from build123d import *

# Parameters (mm, degrees)
BOSS_EXTRUDE1_DEPTH = 5
SKETCH2_W           = 24.8
SKETCH2_H           = 23.2
CUT_EXTRUDE1_DEPTH  = 5
BOSS_EXTRUDE2_START = 5
BOSS_EXTRUDE2_DEPTH = 5
SKETCH4_R           = 1.95
CUT_EXTRUDE2_DEPTH  = 10
CUT_EXTRUDE3_DEPTH  = 5
CUT_EXTRUDE4_DEPTH  = 29.2


with BuildPart() as part:
    # Sketch1 → Boss-Extrude1 (new body)
    with BuildSketch(Plane.XY):
        with BuildLine():
            Line((14.2, 0), (14.2, 5))
            Line((14.2, 5), (50, 5))
            Line((50, 5), (50, -24.2))
            Line((50, -24.2), (-50, -24.2))
            Line((-50, -24.2), (-50, 5))
            Line((-50, 5), (-14.2, 5))
            Line((-14.2, 5), (-14.2, 0))
            ThreePointArc((-14.2, 0), (0, -14.2), (14.2, 0))
        make_face()
        with BuildLine():
            Line((-5, -18.431553888), (5, -18.431553888))
            ThreePointArc((5, -18.431553888), (7, -20.431553888), (5, -22.431553888))
            Line((5, -22.431553888), (-5, -22.431553888))
            ThreePointArc((-5, -22.431553888), (-7, -20.431553888), (-5, -18.431553888))
        make_face(mode=Mode.SUBTRACT)
    extrude(amount=BOSS_EXTRUDE1_DEPTH)

    # Sketch2 → Cut-Extrude1 (cut)
    with BuildSketch(Plane.XY.offset(5)):
        with Locations((-33.6, -9.6)):
            Rectangle(SKETCH2_W, SKETCH2_H)
        with Locations((33.6, -9.6)):
            Rectangle(SKETCH2_W, SKETCH2_H)
    extrude(amount=-CUT_EXTRUDE1_DEPTH, mode=Mode.SUBTRACT)

    # Sketch3 → Boss-Extrude2 (add)
    with BuildSketch(Plane(origin=(0, 0, 0), x_dir=(-1, 0, 0), z_dir=(0, 0, -1)).offset(BOSS_EXTRUDE2_START)):
        with BuildLine():
            Line((-20, 5), (-20, 0))
            ThreePointArc((-20, 0), (-19.267766953, -1.767766953), (-17.5, -2.5))
            Line((-17.5, -2.5), (-13.978197309, -2.5))
            ThreePointArc((-13.978197309, -2.5), (-14.144440636, -1.25491), (-14.2, 0))
            Line((-14.2, 0), (-14.2, 5))
            Line((-14.2, 5), (-20, 5))
        make_face()
        with BuildLine():
            ThreePointArc((14.2, 0), (14.144440636, -1.25491), (13.978197309, -2.5))
            Line((13.978197309, -2.5), (17.5, -2.5))
            ThreePointArc((17.5, -2.5), (19.267766953, -1.767766953), (20, 0))
            Line((20, 0), (20, 5))
            Line((20, 5), (14.2, 5))
            Line((14.2, 5), (14.2, 0))
        make_face()
    extrude(amount=-BOSS_EXTRUDE2_DEPTH)

    # Sketch4 → Cut-Extrude2 (cut)
    with BuildSketch(Plane(origin=(0, 0, -5), x_dir=(-1, 0, 0), z_dir=(0, 0, -1))):
        with Locations((-17.5, 0)):
            Circle(SKETCH4_R)
        with Locations((17.5, 0)):
            Circle(SKETCH4_R)
    extrude(amount=-CUT_EXTRUDE2_DEPTH, mode=Mode.SUBTRACT)

    # Sketch5 → Cut-Extrude3 (cut)
    with BuildSketch(Plane.XY.offset(5)):
        with BuildLine():
            Line((-7.5, -15.547171584), (-7.5, -13.852075657))
            ThreePointArc((-7.5, -13.852075657), (-7.513947323, -13.801135135), (-7.551898734, -13.764404292))
            ThreePointArc((-7.551898734, -13.764404292), (-8.068261954, -13.46822739), (-8.573026316, -13.15268869))
            ThreePointArc((-8.573026316, -13.15268869), (-8.739609576, -12.972022031), (-8.8, -12.733813254))
            Line((-8.8, -12.733813254), (-8.8, -11.099557513))
            Line((-8.8, -11.099557513), (8.8, -11.099557513))
            Line((8.8, -11.099557513), (8.8, -12.733813254))
            ThreePointArc((8.8, -12.733813254), (8.739609576, -12.972022031), (8.573026316, -13.15268869))
            ThreePointArc((8.573026316, -13.15268869), (8.068261954, -13.46822739), (7.551898734, -13.764404292))
            ThreePointArc((7.551898734, -13.764404292), (7.513947323, -13.801135135), (7.5, -13.852075657))
            Line((7.5, -13.852075657), (7.5, -15.547171584))
            ThreePointArc((7.5, -15.547171584), (7.148528137, -16.395699721), (6.3, -16.747171584))
            Line((6.3, -16.747171584), (-6.3, -16.747171584))
            ThreePointArc((-6.3, -16.747171584), (-7.148528137, -16.395699721), (-7.5, -15.547171584))
        make_face()
    extrude(amount=-CUT_EXTRUDE3_DEPTH, mode=Mode.SUBTRACT)

    # Sketch7 → Cut-Extrude4 (cut)
    with BuildSketch(Plane(origin=(0, 5, 0), x_dir=(1, 0, 0), z_dir=(0, 1, 0))):
        with BuildLine():
            Line((49.696579359, 0), (50, 0))
            Line((50, 0), (50, -5))
            Line((50, -5), (49.997973832, -5.049874854))
            ThreePointArc((49.997973832, -5.049874854), (49.911184048, -2.521123203), (49.696579359, 0))
        make_face()
        with BuildLine():
            Line((-50, -5), (-49.997973832, -5.049874854))
            ThreePointArc((-49.997973832, -5.049874854), (-49.911184048, -2.521123203), (-49.696579359, 0))
            Line((-49.696579359, 0), (-50, 0))
            Line((-50, 0), (-50, -5))
        make_face()
    extrude(amount=-CUT_EXTRUDE4_DEPTH, mode=Mode.SUBTRACT)


solid = part.part
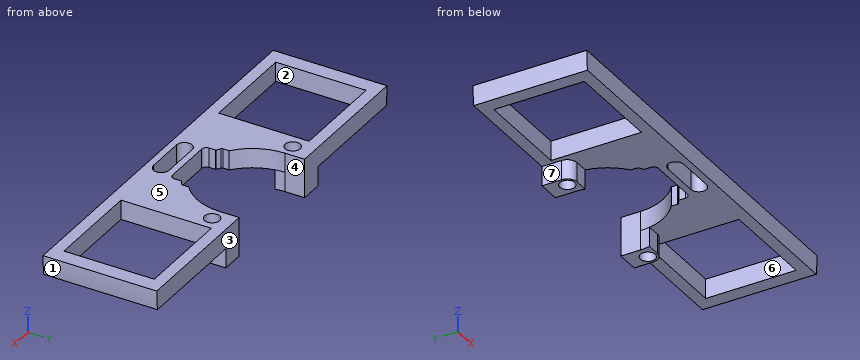
Model file for the job. Use its own axes, mm. Face numbers are marked on the shaded views. A direction names the side the tool comes from. Give positions to 0.01 mm unless a question says otherwise; leave off trailing zeros. Write each loop counter-clockwise with the first axis right and the second up, starting at its lowest first coordinate (ties: lowest second). Pieces come first, ordered by that corner, then holes. Notation, with made-up numbers: M 38,-13.75 L 71,-13.75 A20 ccw 71,25.25 Z; hole C 72,69 d1. An arc over 180 degrees is marked long. One line per item, written item: value. Start each with the question number.
Q1. Saw through at C-C, the plane y = -5. Write the cut outline in (x, z), plus the area to 3 significant figures.
Q2. Saw through at A-A, the plane z = -1.25. Write the cut outline in (x, y), plus the area to 3 significant figures.
Q3. Saw through at B-B, the plane x = -26. Write the cut outline in (y, z).
Q4. 3-axis set-ups, long thin cutter, end or side, ignore diameter. For the marked faces 4, 5, 6 and 7: which of +Z, -Z, +X, -X, +Y, -Y reach the whole face in a straight line?
Q5. Drop flat-ended pins along their axis: pin 1 Ø1.1 at (x, z) = (-15.5, -3) entering from -Y; pin 2 Ø4 at (y, z) = (-13.5, 1.5) entering from +X; pin 3 Ø2.5 at (y, z) = (2.5, -2.5) entering from +X; pin 4 Ø1 at (y, z) = (-14, -1.5) entering from -X. Give the stop position or say it passes through.
Q6. Probe probe 1 along Y at (x, z) = (-17.5, 3.25); probe 2 along X at (y, z) = (3.75, -4.5); probe 3 along X at (y, z) = (-1.5, -3). List the from-to ranges inside material, lowest first. Write a range as [from, to].
Q7. Two-plate mould, pull along X, no slides. Class the marked faces 1, 2 and 3: +X half, -X half, draft (parallel to the pull), parting line (faces both ways), or undercut.
Output values:
1. outline: M -50,5 A50 ccw -49.7,0 L -46,0 L -46,5 Z; M -21.2,0 L -13.29,0 L -13.29,5 L -21.2,5 Z; M 13.29,0 L 21.2,0 L 21.2,5 L 13.29,5 Z; M 46,0 L 49.7,0 A50 ccw 50,5 L 46,5 Z
1. area: 118 mm²
2. outline: M -20,0 A2.5 ccw -17.5,-2.5 L -13.98,-2.5 A14.2 cw -14.2,0 L -14.2,5 L -20,5 Z; M 13.98,-2.5 L 17.5,-2.5 A2.5 ccw 20,0 L 20,5 L 14.2,5 L 14.2,0 A14.2 cw Z; hole C -17.5,0 d3.9; hole C 17.5,0 d3.9
2. area: 60.8 mm²
3. outline: M -24.2,0 L -21.2,0 L -21.2,5 L -24.2,5 Z; M 2,0 L 5,0 L 5,5 L 2,5 Z
4. face 4: +Z, -Z, +Y
4. face 5: +Z, +X, -X, +Y, -Y
4. face 6: +Z, -Z
4. face 7: -Z, -X, +Y, -Y
5. pin 1: stops at y = -2.5
5. pin 2: stops at x = 49.96
5. pin 3: stops at x = 20
5. pin 4: passes through
6. probe 1: y = [-24.2, -1.95], [1.95, 5]
6. probe 2: x = [-20, -14.2], [14.2, 20]
6. probe 3: x = [-19.5, -18.75], [-16.25, -14.12], [14.12, 16.25], [18.75, 19.5]
7. face 1: +X half
7. face 2: undercut
7. face 3: draft
